CAD build for the part. Positions are in the model's coordinates, mm. Round coordinates to 2 decimals unless told otherwise and drop trailing zeros. Write each loop counter-clockwise with the first axis right and the second up, starting at its lowest first coordinate (ties: lowest second). Pieces come first, ordered by that corner, then holes. Notation, with made-up numbers: (42.5, 20) -> (88.5, 20) arc R20 cw to (88.5, 51) -> close; hole circle Ø11 at (-8, 78). An arc over 180 degrees is marked (long way). Put each result on its own line as item: value. Start each with the question number.
1. Saw through at B-B on x = 2. List the corners of the cut face in (y, z) (3 decimals).
2. Flat gauge pins, fed straight in: P1, Ø3, axis at x = 2, z = 116, coming from the -Y side; P2, Ø2, axis at y = -64.5, z = 40, coming from the -X side; P3, Ø3, axis at x = 4.5, y = -42, coming from the +Z side; P4, Ø5.5, axis at y = -25.4, z = 98.425, coming from the -X side. Where does each tip first touch, or does it go through?
3. Saw through at D-D on y = -10.5. List the corners of the cut face in (x, z), and give its area (3 significant figures).
4. Drill centre lines: line 1 (Y direction, x = 2.25, z = 31.75) (3 decimals); line 2 (Y direction, x = 5, z = 97); line 3 (Z direction, x = 3.5, y = -23.5). Where is each one in solid material? Low to high. Write a range as from..to.
5. Pull direction Y, two halves, no side cores. Call faces 1 (the flat face through (3, 0, 81)), 2 (the flat face through (3.131, -48.292, 81.394)), 3 (the cylindrical face through (3.219, -66.177, 33.457)), 4 (the flat face through (6.35, -27, 47)): pulls with the +Y half, pulls with the -Y half, needs draft (parallel to the pull), parting line crosses it, or undercut.
6. Saw through at C-C on y = -25.4. List the corners of the cut face in (x, z), and give its area (3 significant figures).
7. Saw through at A-A on z = 31.75. List the corners of the cut face in (x, y) (3 decimals), and give its area (3 significant figures).
Autodesk Inventor part; units mm, degrees
ref_plane "YZ Plane" through (0, 0, 0) normal (1, 0, 0) x (0, 1, 0)
ref_plane "XZ Plane" through (0, 0, 0) normal (0, 1, 0) x (-1, 0, 0)
ref_plane "XY Plane" through (0, 0, 0) normal (0, 0, 1) x (1, 0, 0)
sketch "Sketch1" plane through (0, 0, 0) normal (1, 0, 0) x (0, 1, 0)
  line L0 (0, 0) -> (0, 165.1)
  line L1 (0, 0) -> (-95.25, 0)
  line L2 (-95.25, 0) -> (0, 165.1)
  dimension "d0" = 165.1
  dimension "d1" = 95.25
extrude "Extrusion1" add sketch "Sketch1" along normal blind 6.35
sketch "Sketch2" plane through (0, 0, 0) normal (-1, 0, 0) x (0, 0, 1)
  line L0 (0, 0) -> (165.1, 0)
  line L1 (0, -95.25) -> (0, 0)
  point P0 (98.425, -25.4)
  point P1 (31.75, -63.5)
  dimension "d4" = 25.4
  dimension "d5" = 98.425
  dimension "d6" = 31.75
  dimension "d7" = 63.5
hole "Hole1" at (0, -25.4, 98.425) at (0, -63.5, 31.75) direction (1, 0, 0) diameter 6.35 end through all
properties part number "30deg gusset plate" material "Aluminum 6061"
Return value:
1. outline: (-95.25, 0) -> (0, 0) -> (0, 165.1) -> close; hole circle Ø6.35 at (-63.5, 31.75); hole circle Ø6.35 at (-25.4, 98.425)
2. P1: stops at y = -29.19
2. P2: stops at x = 0
2. P3: stops at z = 94.9
2. P4: passes through
3. outline: (0, 0) -> (6.35, 0) -> (6.35, 146.9) -> (0, 146.9) -> close
3. area: 933 mm^2
4. line 1: y = -76.933..-66.675, -60.325..0
4. line 2: y = -39.29..-28.24, -22.56..0
4. line 3: z = 0..95.88, 100.97..124.37
5. face 1: pulls with the +Y half
5. face 2: pulls with the -Y half
5. face 3: undercut
5. face 4: needs draft
6. outline: (0, 0) -> (6.35, 0) -> (6.35, 95.25) -> (0, 95.25) -> close; (0, 101.6) -> (6.35, 101.6) -> (6.35, 121.07) -> (0, 121.07) -> close
6. area: 728 mm^2
7. outline: (0, -76.933) -> (6.35, -76.933) -> (6.35, -66.675) -> (0, -66.675) -> close; (0, -60.325) -> (6.35, -60.325) -> (6.35, 0) -> (0, 0) -> close
7. area: 448 mm^2
